Geometry check sheet. Reference: the model listing, model coordinates, mm. Face numbers are marked on the shaded views. Coordinates: 2 decimals unless noted, no trailing zeros. Order: outer loops, then holes, each group sorted by start corner. A loop starts at its lowest first (then second) coordinate and runs counter-clockwise, first axis right, second up. Notation, with made-up numbers: (37.25, 58) - (85.25, 58) arc R33 cw to (85.25, 95) - close; hole circle Ø1 at (55.25, 17.5). An arc over 180 degrees is marked (long way). Return JSON: item names as keys, results as strings. Group by question number.
Item 1: Section check B-B on y = 15.5. Enter the section's corners in (x, z).
Item 2: Draft check along Z on the marked faces 1, 2 and 3. Enter one of: pulls with the +Z half, pulls with the -Z half, needs draft (parallel to the pull), parting line crosses it, or undercut.
Item 3: Section check C-C on x = 53.5. Enter the section's corners in (y, z) (3 decimals).
Item 4: Section check A-A on z = 14. Enter the section's corners in (x, y).
Item 5: Section check D-D on x = -6. Enter the section's corners in (y, z).
Item 6: Gauge pin test, flat ends, axial feed: pin 1 (12 mm diameter, centred on y = 20, z = 18, fed in from +X); pin 2 (8 mm diameter, centred on y = 8, z = 20.5, fed in from -X); pin 3 (1.5 mm diameter, centred on y = 37, z = 10, fed in from -X); pin 4 (0.9 mm diameter, centred on y = 28, z = 1, fed in from +X). Record the tip position at first contact, or that the pin passes through.
Item 7: Scan lines: probe 1 along Z at (x, y) = (24, 12.5); probe 2 along Z at (x, y) = (23.5, 42); probe 3 along Z at (x, y) = (-110, 5.5). Record each from-to range of solid material in increasing order.
from build123d import *

# Parameters (mm, degrees)
SKETCH_1_W      = 200
SKETCH_1_H      = 60
SKETCH_1_R      = 6
EXTRUDE_1_DEPTH = 3
SKETCH_1_3_R    = 6
EXTRUDE_2_DEPTH = 50
SKETCH_2_R      = 26.59997625
SKETCH_2_R_2    = 22.5
EXTRUDE_3_DEPTH = 145


with BuildPart() as part:
    # Sketch 1 → Extrude 1 (new body)
    with BuildSketch(Plane(origin=(-45.881001885, 0, 0), x_dir=(1, 0, 0), z_dir=(0, 0, 1))):
        with Locations((2.697095436, 30)):
            Rectangle(SKETCH_1_W, SKETCH_1_H)
        with Locations((-75.721397193, 30)):
            Circle(SKETCH_1_R, mode=Mode.SUBTRACT)
    extrude(amount=EXTRUDE_1_DEPTH)

    # Sketch 1_3 → Extrude 2 (add)
    with BuildSketch(Plane(origin=(-45.881001885, 0, 0), x_dir=(1, 0, 0), z_dir=(0, 0, 1))):
        with Locations((-75.721397193, 30)):
            Circle(SKETCH_1_3_R)
    extrude(amount=EXTRUDE_2_DEPTH)

    # Sketch 2 → Extrude 3 (add)
    with BuildSketch(Plane(origin=(0, 0, 2.268932334), x_dir=(0, 0, -1), z_dir=(1, 0, 0))):
        with Locations(Location((-26.59997625, 29.77500334, 0), (0, 0, 346.535956225))):
            Circle(SKETCH_2_R)
        with Locations((-26.59997625, 29.77500334)):
            Circle(SKETCH_2_R_2, mode=Mode.SUBTRACT)
    extrude(amount=EXTRUDE_3_DEPTH)


solid = part.part
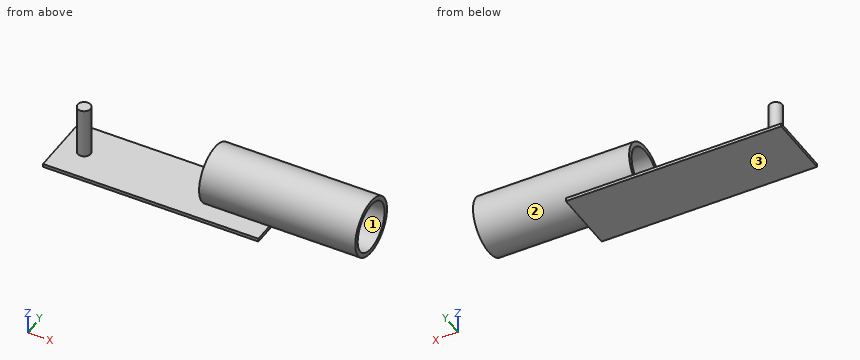
Computed:
{
 "1": {"outline": "(-143.18, 0) - (56.82, 0) - (56.82, 3) - (-143.18, 3) - close; (0, 6.42) - (145, 6.42) - (145, 11.48) - (0, 11.48) - close; (0, 46.26) - (145, 46.26) - (145, 51.31) - (0, 51.31) - close"},
 "2": {"face 1": "undercut", "face 2": "undercut", "face 3": "pulls with the -Z half"},
 "3": {"outline": "(0, 0) - (60, 0) - (60, 3) - (35.968, 3) arc R26.6 ccw (long way) to (23.582, 3) - (0, 3) - close; hole circle Ø45 at (29.775, 28.869)"},
 "4": {"outline": "circle Ø12 at (-121.6, 30); (0, 7.72) - (145, 7.72) - (145, 12.89) - (0, 12.89) - close; (0, 46.66) - (145, 46.66) - (145, 51.83) - (0, 51.83) - close"},
 "5": {"outline": "(0, 0) - (60, 0) - (60, 3) - (0, 3) - close"},
 "6": {"pin 1": "stops at x = -117.13", "pin 2": "stops at x = 0", "pin 3": "passes through", "pin 4": "stops at x = 56.82"},
 "7": {"probe 1": "z = 0 to 3, 8.64 to 14.45, 43.29 to 49.1", "probe 2": "z = 0 to 3, 5.24 to 9.98, 47.76 to 52.49", "probe 3": "z = 0 to 3"}
}
